```python
from build123d import *

# Parameters (mm, degrees)
SKETCH_1_W               = 29
SKETCH_1_H               = 38.5
EXTRUDE_1_DEPTH          = 24
SHELL_1_T                = -1.5
SKETCH_7_W               = 26
SKETCH_7_H               = 5.5
EXTRUDE_7_DEPTH          = 2.5
SKETCH_5_W               = 2.7
SKETCH_5_H               = 1.5
EXTRUDE_8_DEPTH          = 8
SKETCH_6_W               = 2.7
SKETCH_6_H               = 1.5
EXTRUDE_9_DEPTH          = 9
CUT_EXTRUDE_7_DEPTH      = 1.5
SKETCH_9_W               = 29
SKETCH_9_H               = 38.5
EXTRUDE_10_DEPTH         = 0.5
FILLET_3_R               = 2
CUT_EXTRUDE_8_DEPTH      = 1.5
CUT_EXTRUDE_8_DEPTH_BACK = 7
SKETCH_2_W               = 12
SKETCH_2_H               = 2


with BuildPart() as part:
    # 草图1 → 凸台-拉伸1 (new body)
    with BuildSketch(Plane.XY):
        with Locations((14.5, -19.25)):
            Rectangle(SKETCH_1_W, SKETCH_1_H)
    extrude(amount=EXTRUDE_1_DEPTH)

    # 抽壳1
    shell_1_openings = [part.faces().sort_by_distance(p)[0] for p in [
        (14.5, -19.25, 24),
    ]]
    offset(amount=SHELL_1_T, openings=shell_1_openings, kind=Kind.INTERSECTION)

    # 草图7 → 凸台-拉伸7 (add)
    with BuildSketch(Plane.XY.offset(1.5)):
        with Locations((14.5, -34.25)):
            Rectangle(SKETCH_7_W, SKETCH_7_H)
    extrude(amount=EXTRUDE_7_DEPTH)

    # 草图5 → 凸台-拉伸8 (add)
    with BuildSketch(Plane.ZY.offset(-27.5)):
        with Locations((2.85, -2.25)):
            Rectangle(SKETCH_5_W, SKETCH_5_H)
    extrude(amount=EXTRUDE_8_DEPTH)

    # 草图6 → 凸台-拉伸9 (add)
    with BuildSketch(Plane(origin=(1.5, 0, 0), x_dir=(0, 0, -1), z_dir=(1, 0, 0))):
        with Locations((-2.85, -2.25)):
            Rectangle(SKETCH_6_W, SKETCH_6_H)
    extrude(amount=EXTRUDE_9_DEPTH)

    # 草图8 → 切除-拉伸7 (cut)
    with BuildSketch(Plane.ZY):
        with BuildLine():
            Line((19, -21), (19, -21.803847577))
            ThreePointArc((19, -21.803847577), (16, -33), (13, -21.803847577))
            Line((13, -21.803847577), (13, -21))
            ThreePointArc((13, -21), (16, -18), (19, -21))
        make_face()
    extrude(amount=-CUT_EXTRUDE_7_DEPTH, mode=Mode.SUBTRACT)

    # 草图9 → 凸台-拉伸10 (add)
    with BuildSketch(Plane(origin=(0, 0, 0), x_dir=(-1, 0, 0), z_dir=(0, 0, -1))):
        with Locations((-14.5, -19.25)):
            Rectangle(SKETCH_9_W, SKETCH_9_H)
    extrude(amount=EXTRUDE_10_DEPTH)

    # 圆角3
    fillet_3_edges = [part.edges().sort_by_distance(p)[0] for p in [
        (0, 0, 11.75),
        (29, 0, 11.75),
        (29, -38.5, 11.75),
        (0, -38.5, 11.75),
    ]]
    fillet(fillet_3_edges, radius=FILLET_3_R)

    # 草图2 → 切除-拉伸8 (cut, two sides: drawn at the far end of the back side and taken through both)
    with BuildSketch(Plane(origin=(0, 0, 0), x_dir=(-1, 0, 0), z_dir=(0, 0, -1)).offset(-CUT_EXTRUDE_8_DEPTH_BACK)):
        with Locations((-15, -1)):
            Rectangle(SKETCH_2_W, SKETCH_2_H)
    extrude(amount=CUT_EXTRUDE_8_DEPTH + CUT_EXTRUDE_8_DEPTH_BACK, mode=Mode.SUBTRACT)


solid = part.part
```
Read the model definition and answer for the solid it produces. Units are mm, in the model's axes. A direction names the side the tool comes from. Give positions to 0.01 mm unless a question says otherwise; leave off trailing zeros. Order: outer loops, then holes, each group sorted by start corner. A loop starts at its lowest first (then second) coordinate and runs counter-clockwise, first axis right, second up. Notation, with made-up numbers: (-34, 23.25) -> (14, 23.25) arc R30 cw to (14, 58.25) -> close; hole circle Ø7 at (-32, 18.5). An arc over 180 degrees is marked (long way). One line per item, written item: value. Start each with the question number.
(1) The part is cut by section D-D (z = 16). Determine the outline of the cut face in (x, y), and give its area (3 significant figures).
(2) For a pull along Y with two mould halves and no side action, classify faces 5 (the flat face through (0.5, -19.2, 24)), 6 (the cylindrical face through (28.43, -37.9, 11.58)), 7 (the flat face through (6, -3, 3)) as released by +Y, released by -Y, zero draft, split by the parting line, or undercut.
(3) Straight lines are drawn through the part: L1, parallel to X at y = -13, z = 5; L2, parallel to Y at x = 3.75, z = 17; L3, parallel to X at y = -24, z = 14. For each, find the intervals that lie inside material, in ascending order.
(4) Flat-ended cylindrical pins translate along their axes: P1, Ø8, axis at x = 9, y = -17, coming from the +Z side; P2, Ø12, axis at x = 14, z = 3.5, coming from the +Y side; P3, Ø11, axis at y = -27, z = 16, coming from the -X side; P4, Ø4, axis at x = 17.5, z = 1.5, coming from the +Y side. Find the tip coordinate at first contact, or state that the pin passes through.
(5) The part is cut by section A-A (x = 9.5). Determine the outline of the cut face in (y, z).
(6) The part is cut by section C-C (y = -27). Determine the outline of the cut face in (x, z), and give its area (4 significant figures).
(7) A tool of negligible diameter and unlimited length cuts with its end or side. For faces 1 (the flat face through (19.5, -2.5, 2.8)), 2 (the cylindrical face through (1, -18, 16)), 3 (the flat face through (24, -2, 4.2)), 4 (the flat face through (21, -1, 3)), from which of +Z, -Z, +X, -X, +Y, -Y can it reach the whole face along a straight path? Write none if from no direction.
(8) The part is cut by section B-B (z = 9.5). Determine the outline of the cut face in (x, y), and give its area (3 significant figures).
Taken from the geometry:
1. outline: (0, -36.5) arc R2 ccw to (2, -38.5) -> (27, -38.5) arc R2 ccw to (29, -36.5) -> (29, -2) arc R2 ccw to (27, 0) -> (2, 0) arc R2 ccw to (0, -2) -> (0, -18) -> (1.5, -18) -> (1.5, -1.5) -> (27.5, -1.5) -> (27.5, -37) -> (1.5, -37) -> (1.5, -33) -> (0, -33) -> close
1. area: 168 mm^2
2. face 5: zero draft
2. face 6: released by -Y
2. face 7: undercut
3. L1: 0 to 1.5, 27.5 to 29
3. L2: -38.5 to -37, -1.5 to 0
3. L3: 27.5 to 29
4. P1: z = 1.5
4. P2: y = 0
4. P3: x = 27.5
4. P4: y = -2
5. outline: (-38.5, -0.5) -> (-2, -0.5) -> (-2, 4.2) -> (-3, 4.2) -> (-3, 1.5) -> (-31.5, 1.5) -> (-31.5, 4) -> (-37, 4) -> (-37, 24) -> (-38.5, 24) -> close; (-1.5, 7) -> (0, 7) -> (0, 24) -> (-1.5, 24) -> close
6. outline: (0, -0.5) -> (29, -0.5) -> (29, 24) -> (27.5, 24) -> (27.5, 1.5) -> (1.5, 1.5) -> (1.5, 10) -> (0, 10) -> close; (0, 22) -> (1.5, 22) -> (1.5, 24) -> (0, 24) -> close
6. area: 107.5 mm^2
7. face 1: +Z, +Y
7. face 2: -X
7. face 3: +Z
7. face 4: -Z, +Y
8. outline: (0, -36.5) arc R2 ccw to (2, -38.5) -> (27, -38.5) arc R2 ccw to (29, -36.5) -> (29, -2) arc R2 ccw to (27, 0) -> (2, 0) arc R2 ccw to (0, -2) -> close; hole (1.5, -37) -> (27.5, -37) -> (27.5, -1.5) -> (1.5, -1.5) -> close
8. area: 190 mm^2
